Study the drawing (mm; zero at the part's minimum x, y, z) and answer. Give positions to 0.01 mm unless a question says otherwise; leave off trailing zeros. Order: outer loops, then holes, each group sorted by start corner. A loop starts at its lowest first (then second) coordinate and runs counter-clockwise, first axis right, second up. Notation, with made-up numbers: (0, 44) - (35, 44) arc R12 cw to (35, 57) - close; hole circle Ø8 at (-28, 18). An arc over 180 degrees is marked (long way). Write each question's results on one line, items separated by ' | '. Start each with the question number.
1. Section A-A (x = 391.5) is taken. Give the vertices of the cut face in (y, z).
2. Section C-C (z = 58.5) is taken. Give the vertices of the cut face in (x, y), and give its area (3 significant figures).
3. Section B-B (y = 5.75) is taken. Give the vertices of the cut face in (x, z), and give its area (3 significant figures).
4. Find the intervals of material crossed by L1, parallel to X at y = 4.5, z = 18; L2, parallel to X at y = 5.5, z = 62; L3, parallel to Z at x = 117, y = 7, in increasing order.
5. Section D-D (x = 466.5) is taken. Give the vertices of the cut face in (y, z), and give its area (3 significant figures).
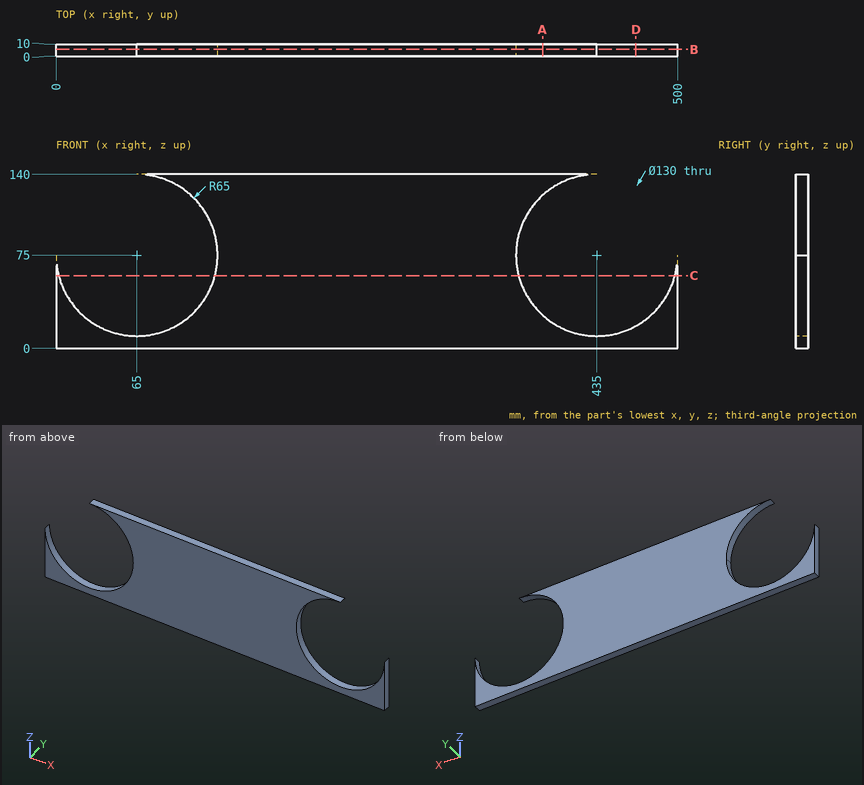
Reported:
1) outline: (0, 0) - (10, 0) - (10, 26.7) - (0, 26.7) - close; (0, 123.3) - (10, 123.3) - (10, 140) - (0, 140) - close
2) outline: (0, 0) - (2.13, 0) - (2.13, 10) - (0, 10) - close; (127.87, 0) - (372.13, 0) - (372.13, 10) - (127.87, 10) - close; (497.87, 0) - (500, 0) - (500, 10) - (497.87, 10) - close | area: 2,490 mm²
3) outline: (0, 0) - (500, 0) - (500, 75) arc R65 cw (long way) to (435, 140) - (65, 140) arc R65 cw (long way) to (0, 75) - close | area: 41,600 mm²
4) L1: 0 to 33.76, 96.24 to 403.76, 466.24 to 500 | L2: 0 to 1.31, 128.69 to 371.31, 498.69 to 500 | L3: 0 to 36, 114 to 140
5) outline: (0, 0) - (10, 0) - (10, 18.14) - (0, 18.14) - close | area: 181 mm²
